Could you check a few things on this model? Use its own coordinates, in mm. A direction names the side the tool comes from. Coordinates: 2 decimals unless noted, no trailing zeros. Order: outer loops, then holes, each group sorted by start corner. A loop starts at its lowest first (then second) coordinate and runs counter-clockwise, first axis right, second up.
```python
from build123d import *

# Parameters (mm, degrees)
BOSS_EXTRUDE1_DEPTH = 403.86
BOSS_EXTRUDE2_DEPTH = 403.86
CUT_EXTRUDE2_START  = 19.05
SKETCH3_R           = 19.091620187
SKETCH3_R_2         = 20.569967825
SKETCH3_R_3         = 20.984373032
CUT_EXTRUDE2_DEPTH  = 481.006463827
CUT_EXTRUDE3_START  = 19.05
SKETCH4_R           = 22.86
CUT_EXTRUDE3_DEPTH  = 481.006463827
CUT_EXTRUDE4_START  = 25.4
CUT_EXTRUDE4_DEPTH  = 353.06
SKETCH7_R           = 6.35
CUT_EXTRUDE8_DEPTH  = 76.2


with BuildPart() as part:
    # Sketch1 → Boss-Extrude1 (new body)
    with BuildSketch(Plane.XY):
        with BuildLine():
            Line((76.2, 0), (76.2, 55.88))
            Line((76.2, 55.88), (115.061446619, 123.19))
            Line((115.061446619, 123.19), (26.161446619, 155.326122142))
            Line((26.161446619, 155.326122142), (6.688356563, 127))
            ThreePointArc((6.688356563, 127), (0, 120.311643437), (-6.688356563, 127))
            Line((-6.688356563, 127), (-26.161446619, 155.326122142))
            Line((-26.161446619, 155.326122142), (-115.061446619, 123.19))
            Line((-115.061446619, 123.19), (-76.2, 55.88))
            Line((-76.2, 55.88), (-76.2, 0))
            Line((-76.2, 0), (76.2, 0))
        make_face()
    extrude(amount=BOSS_EXTRUDE1_DEPTH)

    # Sketch1_2 → Boss-Extrude2 (add)
    with BuildSketch(Plane.XY):
        with BuildLine():
            Line((76.2, 0), (76.2, 55.88))
            Line((76.2, 55.88), (115.061446619, 123.19))
            Line((115.061446619, 123.19), (26.161446619, 155.326122142))
            Line((26.161446619, 155.326122142), (6.688356563, 127))
            ThreePointArc((6.688356563, 127), (0, 120.311643437), (-6.688356563, 127))
            Line((-6.688356563, 127), (-26.161446619, 155.326122142))
            Line((-26.161446619, 155.326122142), (-115.061446619, 123.19))
            Line((-115.061446619, 123.19), (-76.2, 55.88))
            Line((-76.2, 55.88), (-76.2, 0))
            Line((-76.2, 0), (76.2, 0))
        make_face()
    extrude(amount=BOSS_EXTRUDE2_DEPTH)

    # Sketch3 → Cut-Extrude2 (cut, through all)
    with BuildSketch(Plane(origin=(52.682660739, 145.73906954, 0), x_dir=(0.9404411643717996, -0.3399564918559638, 0), z_dir=(0.33995649185596377, 0.9404411643717995, 0)).offset(CUT_EXTRUDE2_START)):
        with Locations((19.043177743, -60.96)):
            Circle(SKETCH3_R)
        with Locations((19.043177743, -172.72)):
            Circle(SKETCH3_R_2)
        with Locations((19.043177743, -284.48)):
            Circle(SKETCH3_R_3)
    extrude(amount=-CUT_EXTRUDE2_DEPTH, mode=Mode.SUBTRACT)

    # Sketch4 → Cut-Extrude3 (cut, through all)
    with BuildSketch(Plane(origin=(-52.682660739, 145.73906954, 0), x_dir=(0.9404411643717996, 0.3399564918559638, 0), z_dir=(-0.33995649185596377, 0.9404411643717995, 0)).offset(CUT_EXTRUDE3_START)):
        with Locations(Location((-19.085280601, -116.840003489, 0), (0, 0, 180))):
            Circle(SKETCH4_R)
        with Locations(Location((-19.085280601, -228.600003489, 0), (0, 0, 180))):
            Circle(SKETCH4_R)
        with Locations(Location((-19.085280601, -340.360003489, 0), (0, 0, 180))):
            Circle(SKETCH4_R)
    extrude(amount=-CUT_EXTRUDE3_DEPTH, mode=Mode.SUBTRACT)

    # Sketch6 → Cut-Extrude4 (cut)
    with BuildSketch(Plane.XY.offset(CUT_EXTRUDE4_START)):
        with BuildLine():
            Line((50.811289955, 0), (-50.811289955, 0))
            Line((-50.811289955, 0), (-50.811289955, 31.75))
            Line((-50.811289955, 31.75), (-26.302401749, 45.819252354))
            ThreePointArc((-26.302401749, 45.819252354), (0, 52.832), (26.302401749, 45.819252354))
            Line((26.302401749, 45.819252354), (50.811289955, 31.75))
            Line((50.811289955, 31.75), (50.811289955, 0))
        make_face()
    extrude(amount=CUT_EXTRUDE4_DEPTH, mode=Mode.SUBTRACT)

    # Sketch7 → Cut-Extrude8 (cut)
    with BuildSketch(Plane.XZ):
        with Locations(Location((-63.5, 391.16, 0), (0, 0, 270))):
            Circle(SKETCH7_R)
        with Locations(Location((63.5, 12.7, 0), (0, 0, 270))):
            Circle(SKETCH7_R)
    extrude(amount=-CUT_EXTRUDE8_DEPTH, mode=Mode.SUBTRACT)


solid = part.part
```
Item 1: I need wall thicknesses on line 1 (X direction, y = 25, z = 12); line 2 (X direction, y = 38.5, z = 391.16); line 3 (Z direction, x = 6, y = 43.5). Which ranges of each line are inside material? Lowest first, please.
Item 2: Suppose I cut it at A-A (z = 72.5). List the corners of the cut face in (x, y) for me.
Item 3: Which directions (+Z, -Z, +X, -X, +Y, -Y) give clear straight access to the entire face, cutting with the end or side of a thin tool? Please do faces 4 (the face through (-76.2, 28, 199)), 5 (the face through (38.39, 38.88, 227.55)), 6 (the face through (0.147, 120.313, 199.103)).
Item 4: Suppose I cut it at C-C (z = 12.7). List the corners of the cut face in (x, y) for me.
Item 5: Suppose I cut it at B-B (x = 0). List the corners of the cut face in (y, z) for me, and give its area (3 significant figures).
Item 6: Suppose I cut it at D-D (y = 38.5). Count the separate pieces of the cut face and the enclosed holes in it, and give its area (3 significant figures).
Item 7: Thinking about a two-plate mould opening in X: for faces 1 (the face through (-52, 0, 199)), 2 (the face through (-70.12, 75.72, 219.84)), 3 (the face through (71.234, 139.033, 199.103)), which applies, +X half, -X half, draft (parallel to the pull), parting line (faces both ways), or undercut?
Item 8: For pin 1 Ø16 at (y, z) = (8.5, 241.5) entering from +X; pin 2 Ø1 at (y, z) = (110.5, 174.5) entering from -X; pin 3 Ø1 at (x, z) = (0.5, 95) entering from +Y, each with a flat end and sliding along its axis, tell me the tip position at first contact or that it passes through.
Geometry results:
1. line 1: x = -76.2 to 57.19, 69.81 to 76.2
1. line 2: x = -76.2 to -69.85, -57.15 to 76.2
1. line 3: z = 0 to 25.4, 378.46 to 403.86
2. outline: (-115.06, 123.19) - (-76.2, 55.88) - (-76.2, 0) - (-50.81, 0) - (-50.81, 31.75) - (-26.3, 45.82) arc R52.83 cw to (21.52, 48.25) - (56.29, 144.44) - (26.16, 155.33) - (6.69, 127) arc R6.69 cw to (-6.69, 127) - (-26.16, 155.33) - close; (48.4, 33.13) - (50.81, 31.75) - (50.81, 0) - (76.2, 0) - (76.2, 55.88) - (115.06, 123.19) - (84.89, 134.09) - close
3. face 4: +Z, -Z, -X, -Y
3. face 5: -Y
3. face 6: +Z, -Z, +Y
4. outline: (-115.06, 123.19) - (-76.2, 55.88) - (-76.2, 0) - (57.15, 0) - (57.15, 76.2) - (69.85, 76.2) - (69.85, 0) - (76.2, 0) - (76.2, 55.88) - (115.06, 123.19) - (26.16, 155.33) - (6.69, 127) arc R6.69 cw to (-6.69, 127) - (-26.16, 155.33) - close
5. outline: (0, 0) - (120.31, 0) - (120.31, 403.86) - (0, 403.86) - (0, 378.46) - (52.83, 378.46) - (52.83, 25.4) - (0, 25.4) - close
5. area: 29,900 mm2
6. separate pieces: 1
6. enclosed holes: 3
6. area: 30,300 mm2
7. face 1: draft
7. face 2: undercut
7. face 3: +X half
8. pin 1: stops at x = 76.2
8. pin 2: stops at x = -108.02
8. pin 3: stops at y = 120.39
